```python
from build123d import *

# Parameters (mm, degrees)
SKETCH1_R           = 7.5
BOSS_EXTRUDE1_DEPTH = 6.35
SKETCH2_R           = 4.7625
CUT_EXTRUDE1_DEPTH  = 12.7
SKETCH3_R           = 10
SKETCH3_R_2         = 4.7625
BOSS_EXTRUDE2_DEPTH = 3


with BuildPart() as part:
    # Sketch1 → Boss-Extrude1 (new, symmetric)
    with BuildSketch(Plane.XY):
        Circle(SKETCH1_R)
    extrude(amount=BOSS_EXTRUDE1_DEPTH, both=True)

    # Sketch2 → Cut-Extrude1 (cut)
    with BuildSketch(Plane.XY.offset(6.35)):
        Circle(SKETCH2_R)
    extrude(amount=-CUT_EXTRUDE1_DEPTH, mode=Mode.SUBTRACT)

    # Sketch3 → Boss-Extrude2 (add)
    with BuildSketch(Plane.XY.offset(6.35)):
        Circle(SKETCH3_R)
        Circle(SKETCH3_R_2, mode=Mode.SUBTRACT)
    extrude(amount=-BOSS_EXTRUDE2_DEPTH)


solid = part.part
```
Part model, mm, in its own coordinate system. A direction names the side the tool comes from. Round coordinates to 2 decimals unless told otherwise and drop trailing zeros. Write each loop counter-clockwise with the first axis right and the second up, starting at its lowest first coordinate (ties: lowest second). Pieces come first, ordered by that corner, then holes. Notation, with made-up numbers: M -5.5,-9 L 25.5,-9 A9 cw 25.5,-1 Z; hole C 79,71.25 d10. An arc over 180 degrees is marked long. Answer as CSV lines item,"result". Start each with the question number.
1) Drop flat-ended pins along their axis: pin 1 (3 mm diameter, centred on x = -6, z = 2, fed in from -Y); pin 2 (5.5 mm diameter, centred on x = 0, y = 0, fed in from +Z). Give the stop position or say it passes through.
2) Band-saw the part on A-A (y = 0). List the corners of the cut face in (x, z), then the cut area to 3 significant figures.
3) Band-saw the part on C-C (z = -0.75). List the corners of the cut face in (x, y) (1 decimal), then the cut area to 3 significant figures.
4) Mould opens along Y. For faces 3 (the face through (-3.78, -2.9, 0.09)), 4 (the face through (-2.17, -9.76, 4.87)), 5 (the face through (4, 7, 3.35)) say: +Y half, -Y half, draft (parallel to the pull), parting line (faces both ways), or undercut.
5) Band-saw the part on D-D (x = -6). List the corners of the cut face in (y, z), then the cut area to 3 significant figures.
6) Drill centre lines: L1, parallel to Y at x = 0, z = 0.25; L2, parallel to X at y = 1.5, z = -4.5; L3, parallel to Z at x = -3.5, y = 7.5. Where is each one in solid material? Low to high.
7) Which spindle directions (+Z, -Z, +X, -X, +Y, -Y) get a long thin tool onto all of the face, cutting with end or side? Do faces 1 (the face through (-2.4, -4.3, 6.35)), 2 (the face through (-7.493, 0.33, -1.432)). Say none if no direction does.
Worked out:
1,pin 1,"y = -8.45"
1,pin 2,"through"
2,outline,"M -10,3.35 L -7.5,3.35 L -7.5,-6.35 L -4.76,-6.35 L -4.76,6.35 L -10,6.35 Z; M 4.76,-6.35 L 7.5,-6.35 L 7.5,3.35 L 10,3.35 L 10,6.35 L 4.76,6.35 Z"
2,area,"84.5 mm²"
3,outline,"C 0,0 d15; hole C 0,0 d9.5"
3,area,"105 mm²"
4,face 3,"undercut"
4,face 4,"parting line"
4,face 5,"draft"
5,outline,"M -8,3.35 L -4.5,3.35 L -4.5,-6.35 L 4.5,-6.35 L 4.5,3.35 L 8,3.35 L 8,6.35 L -8,6.35 Z"
5,area,"135 mm²"
6,L1,"-7.5 to -4.76, 4.76 to 7.5"
6,L2,"-7.35 to -4.52, 4.52 to 7.35"
6,L3,"3.35 to 6.35"
7,face 1,"+Z, +X, -X, +Y, -Y"
7,face 2,"-Z"
